Autodesk Inventor part; units mm, degrees
ref_plane "YZ Plane" through (0, 0, 0) normal (1, 0, 0) x (0, 1, 0)
ref_plane "XZ Plane" through (0, 0, 0) normal (0, 1, 0) x (-1, 0, 0)
ref_plane "XY Plane" through (0, 0, 0) normal (0, 0, 1) x (1, 0, 0)
sketch "Sketch3" plane through (0, 0, 0) normal (0, 0, 1) x (1, 0, 0)
  line L0 (-15.7, -16.7) -> (15.7, -16.7)
  line L1 (16.7, -15.7) -> (16.7, 15.7)
  line L2 (15.7, 16.7) -> (-15.7, 16.7)
  line L3 (-16.7, 15.7) -> (-16.7, -15.7)
  line L4 (-16.7, -16.7) -> (16.7, 16.7) construction
  line L5 (16.7, -16.7) -> (-16.7, 16.7) construction
  line L6 (-15.7, 16.7) -> (-16.7, 15.7)
  line L7 (15.7, 16.7) -> (16.7, 15.7)
  line L8 (16.7, -15.7) -> (15.7, -16.7)
  line L9 (-16.7, -15.7) -> (-15.7, -16.7)
  line L10 (-4.9497, -8.8994) -> (4.9497, -8.8994)
  line L11 (4.9497, -8.8994) -> (4.9497, 8.8994)
  line L12 (4.9497, 8.8994) -> (-4.9497, 8.8994)
  line L13 (-4.9497, 8.8994) -> (-4.9497, -8.8994)
  line L14 (-4.9497, -8.8994) -> (4.9497, 8.8994) construction
  line L15 (4.9497, -8.8994) -> (-4.9497, 8.8994) construction
  circle A0 centre (-12.14, 12.625) radius 2.045
  circle A1 centre (12.14, 12.625) radius 2.045
  line L16 (0, -16.7) -> (0, 16.7) construction
  circle A2 centre (-12.14, -12.625) radius 2.045
  circle A3 centre (12.14, -12.625) radius 2.045
  line L17 (12.14, 12.625) -> (-12.14, 12.625) construction
  line L18 (-12.14, 12.625) -> (-12.14, -12.625) construction
  line L19 (-12.14, -12.625) -> (12.14, -12.625) construction
  line L20 (12.14, -12.625) -> (12.14, 12.625) construction
  line L21 (-16.7, 0) -> (16.7, 0) construction
  point P0 (0, 0)
  point P1 (0, 0)
  dimension "d0" = 33.4
  dimension "d1" = 33.4
  dimension "d2" = 1
  dimension "d3" = 1
  dimension "d4" = 1
  dimension "d5" = 1
  dimension "d6" = 1
  dimension "d7" = 1
  dimension "d8" = 1
  dimension "d9" = 1
  dimension "d10" = 9.8994
  dimension "d11" = 17.7988
  dimension "d12" = 4.09
  dimension "d13" = 4.09
  dimension "d17" = 4.09
  dimension "d19" = 24.28
  dimension "d20" = 25.25
  dimension "d21" = 4.09
  dimension "d22" = 12.625
  dimension "d23" = 12.14
extrude "Extrusion1" add sketch "Sketch3" along normal blind 4.1
sketch "Sketch6" plane through (0, 0, 4.1) normal (0, 0, 1) x (1, 0, 0)
  line L0 (9, 7.1589) -> (9, -7.1589)
  line L1 (-9, -7.1589) -> (-9, 7.1589)
  arc A0 (-9, -7.1589) -> (9, -7.1589) centre (0, 0) ccw
  arc A1 (9, 7.1589) -> (-9, 7.1589) centre (0, 0) ccw
  dimension "d66" = 18
  dimension "d67" = 11.5
  dimension "d68" = 11.5
  dimension "d69" = 9
extrude "Extrusion4" add sketch "Sketch6" along normal blind 21
sketch "Sketch7" plane through (9, -7.1589, 4.1) normal (1, 0, 0) x (0, 0, -1)
  circle A0 centre (-14, 7.3314) radius 4
  line L0 (-21, 0) -> (-21, 14.3178)
  point P0 (4.1, 7.1589)
  dimension "d58" = 8
  dimension "d59" = 7
extrude "Extrusion5" add sketch "Sketch7" along normal blind 23.5
sketch "Sketch8" plane through (-9, -7.1589, 4.1) normal (-1, 0, 0) x (0, 0, 1)
  circle A0 centre (14, 7.3314) radius 4
  line L0 (21, 14.3178) -> (21, 0)
  point P0 (-4.1, 7.1589)
  dimension "d62" = 8
  dimension "d63" = 7
extrude "Extrusion6" add sketch "Sketch8" along normal blind 23.5
equation "\"d3\" = d2"
equation "\"d5\" = d4"
equation "\"d6\" = d4"
equation "\"d7\" = d6"
equation "\"d8\" = d4"
equation "\"d9\" = d8"
properties part number "coaxToWaveguidWG18" material "Brass, Soft Yellow"
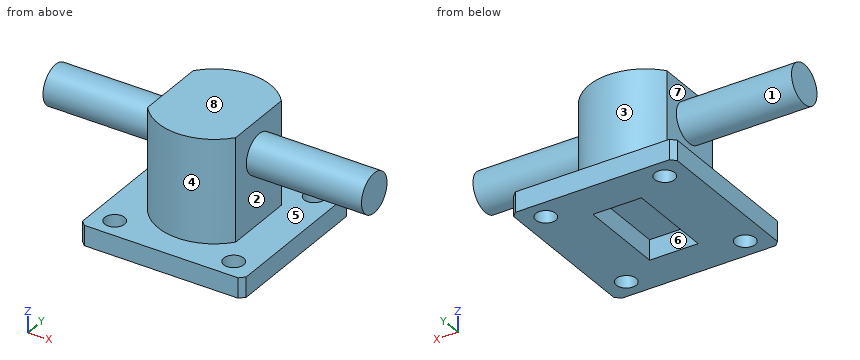
Source: CAD feature listing. Evaluate the final solid. Frame: model axes, mm. Face numbers are marked on the shaded views. A direction names the side the tool comes from. Coordinates: 2 decimals unless noted, no trailing zeros. Loops run counter-clockwise (first coordinate to the right, second up) from the corner with the lowest first, then second, coordinate; pieces in that order, holes last. Notation, with made-up numbers: (40.5, -38.5) - (75.5, -38.5) arc R29 cw to (75.5, -14.5) - close; hole circle Ø3 at (-12, -28). An arc over 180 degrees is marked (long way). Answer as CSV lines item,"result".
1. Ray query, line 1 (Y direction, x = 12.14, z = 2.35); line 2 (X direction, y = -1.5, z = 2); line 3 (Z direction, x = -2, y = -6.5). Return the intervals inside material, ascending.
Established:
line 1,"y = -16.7 to -14.67, -10.58 to 10.58, 14.67 to 16.7"
line 2,"x = -16.7 to -4.95, 4.95 to 16.7"
line 3,"z = 4.1 to 25.1"
2. Section B-B (y = -0.5). Return loops of the section in (x, z).
Established:
outline,"(-32.5, 14.16) - (-9, 14.16) - (-9, 4.1) - (-16.7, 4.1) - (-16.7, 0) - (-4.95, 0) - (-4.95, 4.1) - (4.95, 4.1) - (4.95, 0) - (16.7, 0) - (16.7, 4.1) - (9, 4.1) - (9, 14.16) - (32.5, 14.16) - (32.5, 22.04) - (9, 22.04) - (9, 25.1) - (-9, 25.1) - (-9, 22.04) - (-32.5, 22.04) - close"
3. Mould query, pull axis X, two halves, no side actions, for the marked faces 6, 7 and 8. Classes: released by +X, released by -X, zero draft, split by the parting line, or undercut.
Established:
face 6,"undercut"
face 7,"released by -X"
face 8,"zero draft"
4. Section C-C (z = 15). Return loops of the section in (x, y), then the cut area to 3 significant figures.
Established:
outline,"(-32.5, -2.36) - (-9, -2.36) - (-9, -7.16) arc R11.5 ccw to (9, -7.16) - (9, -2.36) - (32.5, -2.36) - (32.5, 2.7) - (9, 2.7) - (9, 7.16) arc R11.5 ccw to (-9, 7.16) - (-9, 2.7) - (-32.5, 2.7) - close"
area,"604 mm2"
5. Section D-D (x = -15). Return loops of the section in (y, z).
Established:
outline,"(-16.7, 0) - (16.7, 0) - (16.7, 4.1) - (-16.7, 4.1) - close; circle Ø8 at (0.17, 18.1)"
6. Contact query for flat-ended pins moving along their axis: pin 1 (3.5 mm diameter, centred on y = 4, z = 2.5, fed in from -X); pin 2 (2 mm diameter, centred on y = 2.5, z = 2, fed in from +X); pin 3 (3.5 mm diameter, centred on x = 12.14, y = 12.625, fed in from +Z); pin 4 (5.5 mm diameter, centred on x = -12.14, y = 12.625, fed in from +Z). Output: stop coordinate, or through.
Established:
pin 1,"stops at x = -16.7"
pin 2,"stops at x = 16.7"
pin 3,"passes through"
pin 4,"stops at z = 4.1"
7. Reachability of the marked faces 1, 2, 3, 4 and 5 from +Z, -Z, +X, -X, +Y, -Y: full face, straight path, thin tool, end or side. Return the list, or none.
Established:
face 1,"-X"
face 2,"+X"
face 3,"+Z, +Y"
face 4,"+Z, -Y"
face 5,"none"
8. Section A-A (x = 12.14). Return loops of the section in (y, z), then the cut area to 3 significant figures.
Established:
outline,"(-16.7, 0) - (-14.67, 0) - (-14.67, 4.1) - (-16.7, 4.1) - close; (-10.58, 0) - (10.58, 0) - (10.58, 4.1) - (-10.58, 4.1) - close; circle Ø8 at (0.17, 18.1); (14.67, 0) - (16.7, 0) - (16.7, 4.1) - (14.67, 4.1) - close"
area,"154 mm2"
